Here's the drawing with two shaded views (mm, measured from the low corner). I have some questions. A direction names the side the tool comes from. Give positions to 0.01 mm unless a question says otherwise; leave off trailing zeros. Loops run counter-clockwise (first coordinate to the right, second up) from the corner with the lowest first, then second, coordinate; pieces in that order, holes last.
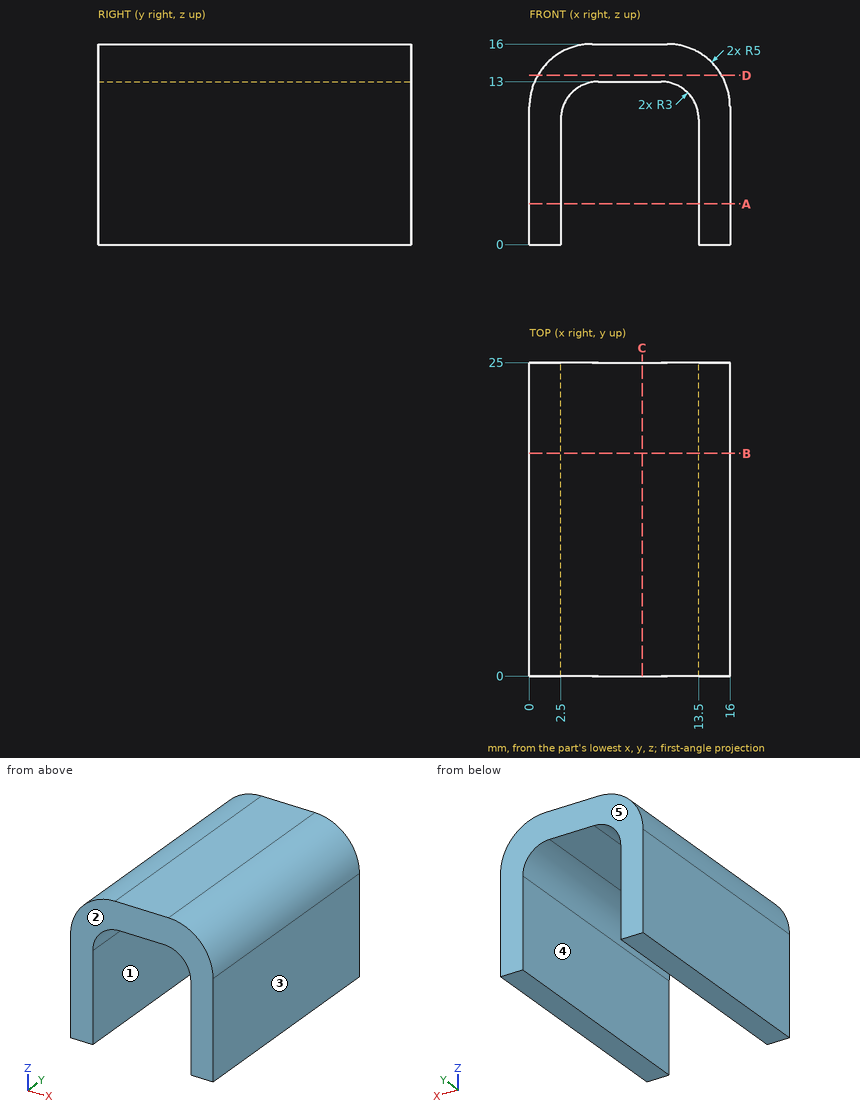
(1) Please list where these lines run through material, in increasing order: probe 1 along X at (y, z) = (3, 5); probe 2 along Z at (x, y) = (8.75, 11.5); probe 3 along X at (y, z) = (8.5, 12.75).
Returned:
probe 1: x = 0 to 2.5, 13.5 to 16
probe 2: z = 13 to 16
probe 3: x = 0.32 to 4.3, 11.7 to 15.68
(2) Suppose I cut it at B-B on y = 17.75. List the corners of the cut face in (x, z) for me.
Returned:
outline: (0, 0) - (2.5, 0) - (2.5, 10) arc R3 cw to (5.5, 13) - (10.5, 13) arc R3 cw to (13.5, 10) - (13.5, 0) - (16, 0) - (16, 11) arc R5 ccw to (11, 16) - (5, 16) arc R5 ccw to (0, 11) - close
(3) Suppose I cut it at D-D on z = 13.5. List the corners of the cut face in (x, y) for me, plus the area to 3 significant figures.
Returned:
outline: (0.67, 0) - (15.33, 0) - (15.33, 25) - (0.67, 25) - close
area: 367 mm2
(4) Which directions (+Z, -Z, +X, -X, +Y, -Y) give clear straight access to the entire face, cutting with the end or side of a thin tool? Please do the marked faces 1 and 2.
Returned:
face 1: -Z, +Y, -Y
face 2: +Z, -Z, +X, -X, -Y
(5) Suppose I cut it at C-C on x = 9. List the corners of the cut face in (y, z) for me, plus the area to 3 significant figures.
Returned:
outline: (0, 13) - (25, 13) - (25, 16) - (0, 16) - close
area: 75.0 mm2
(6) Will these pins go through, and if not, where does the flat tip stop? P1, Ø4, axis at x = 7, y = 10.5, coming from the -Z side; P2, Ø3, axis at x = 11, z = 11.5, coming from the -Y side.
Returned:
P1: stops at z = 12.96
P2: stops at y = 0
(7) Thinking about a two-plate mould opening in X: for the marked faces 3, 4 and 5, which applies, pulls with the +X half, pulls with the -X half, needs draft (parallel to the pull), parting line crosses it, or undercut?
Returned:
face 3: pulls with the +X half
face 4: undercut
face 5: needs draft
(8) Suppose I cut it at A-A on z = 3.25. List the corners of the cut face in (x, y) for me.
Returned:
outline: (0, 0) - (2.5, 0) - (2.5, 25) - (0, 25) - close; (13.5, 0) - (16, 0) - (16, 25) - (13.5, 25) - close
